The listing builds one solid part. Answer for the finished solid, in the listing's coordinates (mm). A direction names the side the tool comes from. Round coordinates to 2 decimals unless told otherwise and drop trailing zeros. Write each loop counter-clockwise with the first axis right and the second up, starting at its lowest first coordinate (ties: lowest second). Pieces come first, ordered by that corner, then holes. Notation, with made-up numbers: (-3, -30) - (44, -30) arc R28 cw to (44, 5) - close; hole circle Ø6 at (32, 72). An arc over 180 degrees is marked (long way). Use a Markdown table: item, result. Add a question column.
1) A cutting plane is placed at D-D (x = -5). Give the vertices of the cut face in (y, z).
2) A tool of negligible diameter and unlimited length cuts with its end or side. For faces 1 (the flat face through (0, 45, 19)), 2 (the cylindrical face through (-14.133, 16.832, -19.507)), from which of +Z, -Z, +X, -X, +Y, -Y can it reach the whole face along a straight path? Write none if from no direction.
3) A cutting plane is placed at A-A (y = 8.5). Give the vertices of the cut face in (x, z).
4) Find the intervals of material crossed by probe 1 along X at (y, z) = (69, 19.4); probe 2 along Z at (x, y) = (18, 78); probe 3 along Y at (x, z) = (-13, -9), in increasing order. Write a range as from..to.
5) A cutting plane is placed at C-C (x = 15). Give the vertices of the cut face in (y, z).
6) Each of these flat-tipped pins is pushed along its axis until it touches: P1, Ø10, axis at x = 11.5, y = 79.5, coming from the -Z side; P2, Ø6.5, axis at x = -17.32, y = 69, coming from the +Z side; P3, Ø1.5, axis at x = 18, z = 10.5, coming from the +Y side; P4, Ø2, axis at x = -10.5, y = 19, coming from the +Z side. Where does it stop, or does it pass through?
7) A cutting plane is placed at B-B (y = 79). State how many separate pieces and enclosed holes the cut face has, then the cut area to 3 significant figures.
8) Determine the mould class of faces 3 (the flat face through (0, 45, -19)), 4 (the flat face through (30, 29.1, -19.2)), 5 (the cylindrical face through (0.867, 82.905, 19.507)) for opening direction X: +X half, -X half, draft (parallel to the pull), parting line (faces both ways), or undercut.
```python
from build123d import *

# Parameters (mm, degrees)
CROQUIS1_W                       = 60
CROQUIS1_H                       = 40
BRIDA_BASE2_DEPTH                = 1
BRIDA_DE_ARISTA1_STRIP_W         = 5.4732
BRIDA_DE_ARISTA1_STRIP_H         = 1
BRIDA_DE_ARISTA1_STRIP_CUT_DEPTH = 60
BRIDA_DE_ARISTA1_DEPTH           = 60
BRIDA_DE_ARISTA2_STRIP_W         = 5.4732
BRIDA_DE_ARISTA2_STRIP_H         = 1
BRIDA_DE_ARISTA2_STRIP_CUT_DEPTH = 60
BRIDA_DE_ARISTA2_DEPTH           = 60
CROQUIS17_R                      = 4
CORTAR_EXTRUIR1_DEPTH            = 50
CROQUIS18_R                      = 4
CORTAR_EXTRUIR2_DEPTH            = 10
CROQUIS19_R                      = 8.95
CORTAR_EXTRUIR3_DEPTH            = 1
CORTAR_EXTRUIR3_DRAFT            = -45
CORTAR_EXTRUIR3_PROFILE_2_DEPTH  = 1
CORTAR_EXTRUIR3_PROFILE_2_DRAFT  = -45


# Sheet-metal steps are written as plain solids
with BuildPart() as part:
    # Croquis1 → Brida base2 (new body)
    with BuildSketch(Plane(origin=(0, 0, 0), x_dir=(1, 0, 0), z_dir=(0, 1, 0))):
        Rectangle(CROQUIS1_W, CROQUIS1_H)
    extrude(amount=-BRIDA_BASE2_DEPTH)

    # Brida de arista1 strip (across the edge) → Brida de arista1 strip cut (cut)
    with BuildSketch(Plane(origin=(-30, 0, 20), x_dir=(0, 0, -1), z_dir=(1, 0, 0))):
        with Locations((-1, -0.5)):
            Rectangle(BRIDA_DE_ARISTA1_STRIP_W, BRIDA_DE_ARISTA1_STRIP_H)
    extrude(amount=BRIDA_DE_ARISTA1_STRIP_CUT_DEPTH, mode=Mode.SUBTRACT)

    # Brida de arista1 section (across the edge) → Brida de arista1 (add)
    with BuildSketch(Plane(origin=(-30, 0, 20), x_dir=(0, 0, -1), z_dir=(1, 0, 0))):
        with BuildLine():
            Line((0, 0.7366), (0, 89))
            Line((0, 89), (1, 89))
            Line((1, 89), (1, 0.7366))
            ThreePointArc((1, 0.7366), (1.215745145, 0.215745145), (1.7366, 0))
            Line((1.7366, 0), (1.7366, -1))
            ThreePointArc((1.7366, -1), (0.508638364, -0.491361636), (0, 0.7366))
        make_face()
    extrude(amount=BRIDA_DE_ARISTA1_DEPTH)

    # Brida de arista2 strip (across the edge) → Brida de arista2 strip cut (cut)
    with BuildSketch(Plane(origin=(30, 0, -20), x_dir=(0, 0, 1), z_dir=(-1, 0, 0))):
        with Locations((-1, -0.5)):
            Rectangle(BRIDA_DE_ARISTA2_STRIP_W, BRIDA_DE_ARISTA2_STRIP_H)
    extrude(amount=BRIDA_DE_ARISTA2_STRIP_CUT_DEPTH, mode=Mode.SUBTRACT)

    # Brida de arista2 section (across the edge) → Brida de arista2 (add)
    with BuildSketch(Plane(origin=(30, 0, -20), x_dir=(0, 0, 1), z_dir=(-1, 0, 0))):
        with BuildLine():
            Line((0, 0.7366), (0, 89))
            Line((0, 89), (1, 89))
            Line((1, 89), (1, 0.7366))
            ThreePointArc((1, 0.7366), (1.215745145, 0.215745145), (1.7366, 0))
            Line((1.7366, 0), (1.7366, -1))
            ThreePointArc((1.7366, -1), (0.508638364, -0.491361636), (0, 0.7366))
        make_face()
    extrude(amount=BRIDA_DE_ARISTA2_DEPTH)

    # Croquis17 → Cortar-Extruir1 (cut)
    with BuildSketch(Plane.XY.offset(20)):
        with BuildLine():
            ThreePointArc((-7.5e-08, 89), (21.213203409, 80.213203462), (30, 59))
            Line((30, 59), (30, 89))
            Line((30, 89), (-7.5e-08, 89))
        make_face()
        with BuildLine():
            ThreePointArc((-30, 59), (-21.213203462, 80.213203409), (-7.5e-08, 89))
            Line((-7.5e-08, 89), (-30, 89))
            Line((-30, 89), (-30, 59))
        make_face()
        with Locations(Location((0, 59, 0), (0, 0, 180))):
            Circle(CROQUIS17_R)
        with Locations(Location((20, 59, 0), (0, 0, 180))):
            Circle(CROQUIS17_R)
        with Locations(Location((10, 76.320508076, 0), (0, 0, 180))):
            Circle(CROQUIS17_R)
        with Locations(Location((17.320508076, 69, 0), (0, 0, 180))):
            Circle(CROQUIS17_R)
        with Locations(Location((0, 79, 0), (0, 0, 180))):
            Circle(CROQUIS17_R)
        with Locations(Location((-10, 76.320508076, 0), (0, 0, 180))):
            Circle(CROQUIS17_R)
        with Locations(Location((-17.320508076, 69, 0), (0, 0, 180))):
            Circle(CROQUIS17_R)
        with Locations(Location((-20, 59, 0), (0, 0, 180))):
            Circle(CROQUIS17_R)
    extrude(amount=-CORTAR_EXTRUIR1_DEPTH, mode=Mode.SUBTRACT)

    # Croquis18 → Cortar-Extruir2 (cut)
    with BuildSketch(Plane(origin=(0, 0, -20), x_dir=(-1, 0, 0), z_dir=(0, 0, -1))):
        with Locations((-15, 20.7366)):
            Circle(CROQUIS18_R)
        with Locations((15, 20.7366)):
            Circle(CROQUIS18_R)
    extrude(amount=-CORTAR_EXTRUIR2_DEPTH, mode=Mode.SUBTRACT)


with BuildPart() as cortar_extruir3_tool:
    # Croquis19 → Cortar-Extruir3 (with draft: the straight prism first)
    with BuildSketch(Plane.XY.offset(20)):
        with Locations((-15, 20.7366)):
            Circle(CROQUIS19_R)
    extrude(amount=-CORTAR_EXTRUIR3_DEPTH)
    # Cortar-Extruir3: the draft: its side faces are tilted about the plane it starts from
    cortar_extruir3_sides = [cortar_extruir3_tool.faces().sort_by_distance(p)[0] for p in [
        (-23.95, 20.7366, 19.5),
    ]]
    draft(cortar_extruir3_sides, Plane.XY.offset(20), CORTAR_EXTRUIR3_DRAFT)


with BuildPart() as part_1:
    add(part.part)

    # Cortar-Extruir3: cut by cortar_extruir3_tool
    add(cortar_extruir3_tool.part, mode=Mode.SUBTRACT)


with BuildPart() as cortar_extruir3_profile_2_tool:
    # Croquis19 → Cortar-Extruir3 profile 2 (with draft: the straight prism first)
    with BuildSketch(Plane.XY.offset(20)):
        with Locations((15, 20.7366)):
            Circle(CROQUIS19_R)
    extrude(amount=-CORTAR_EXTRUIR3_PROFILE_2_DEPTH)
    # Cortar-Extruir3 profile 2: the draft: its side faces are tilted about the plane it starts from
    cortar_extruir3_profile_2_sides = [cortar_extruir3_profile_2_tool.faces().sort_by_distance(p)[0] for p in [
        (6.05, 20.7366, 19.5),
    ]]
    draft(cortar_extruir3_profile_2_sides, Plane.XY.offset(20), CORTAR_EXTRUIR3_PROFILE_2_DRAFT)


with BuildPart() as part_2:
    add(part_1.part)

    # Cortar-Extruir3 profile 2: cut by cortar_extruir3_profile_2_tool
    add(cortar_extruir3_profile_2_tool.part, mode=Mode.SUBTRACT)


solid = part_2.part
```
Entries:
| question | item | result |
|---|---|---|
| 1 | outline | (-1, -18.26) arc R1.74 ccw to (0.74, -20) - (88.58, -20) - (88.58, -19) - (0.74, -19) arc R0.74 cw to (0, -18.26) - (0, 18.26) arc R0.74 cw to (0.74, 19) - (88.58, 19) - (88.58, 20) - (0.74, 20) arc R1.74 ccw to (-1, 18.26) - close |
| 2 | face 1 | +X, -X, +Y |
| 2 | face 2 | +Z, -Z |
| 3 | outline | (-30, -20) - (30, -20) - (30, -19) - (-30, -19) - close; (-30, 19) - (30, 19) - (30, 20) - (-30, 20) - close |
| 4 | probe 1 | x = -28.28..-21.32, -13.32..13.32, 21.32..28.28 |
| 4 | probe 2 | z = -20..-19, 19..20 |
| 4 | probe 3 | y = -1..0 |
| 5 | outline | (-1, -18.26) arc R1.74 ccw to (0.74, -20) - (16.74, -20) - (16.74, -19) - (0.74, -19) arc R0.74 cw to (0, -18.26) - (0, 18.26) arc R0.74 cw to (0.74, 19) - (12.79, 19) - (11.79, 20) - (0.74, 20) arc R1.74 ccw to (-1, 18.26) - close; (24.74, -20) - (65.74, -20) - (65.74, -19) - (24.74, -19) - close; (28.69, 19) - (65.74, 19) - (65.74, 20) - (29.69, 20) - close; (72.26, -20) - (84.98, -20) - (84.98, -19) - (72.26, -19) - close; (72.26, 19) - (84.98, 19) - (84.98, 20) - (72.26, 20) - close |
| 6 | P1 | stops at z = -20 |
| 6 | P2 | passes through |
| 6 | P3 | stops at y = 0 |
| 6 | P4 | stops at z = -19 |
| 7 | separate pieces | 8 |
| 7 | enclosed holes | 0 |
| 7 | area | 49.7 mm² |
| 8 | face 3 | draft |
| 8 | face 4 | +X half |
| 8 | face 5 | undercut |
